```python
from build123d import *

# Parameters (mm, degrees)
F0_R      = 4
F1_DEPTH  = 4
F2_R      = 14.5
F3_DEPTH  = 2
F4_R      = 5
F5_DEPTH  = 1
F3_FACE_R = 14.5
F6_DEPTH  = 2.54


with BuildPart() as f1:
    # F0 (on Top) → F1 (new body)
    with BuildSketch(Plane.XY):
        Circle(F0_R)
    extrude(amount=F1_DEPTH)

    # F2 (on Top) → F3 (join)
    with BuildSketch(Plane.XY):
        Circle(F2_R)
    extrude(amount=-F3_DEPTH)

    # F4 (on Top) → F5 (join)
    with BuildSketch(Plane.XY):
        Circle(F4_R)
    extrude(amount=F5_DEPTH)

    # F3_face (on face) → F6 (join)
    with BuildSketch(Plane(origin=(0, 0, -2), x_dir=(1, 0, 0), z_dir=(0, 0, -1))):
        Circle(F3_FACE_R)
    extrude(amount=F6_DEPTH)


solid = f1.part
```
Build history of the part. All positions in model axes, mm. A direction names the side the tool comes from. Coordinates: 2 decimals unless noted, no trailing zeros. Order: outer loops, then holes, each group sorted by start corner. A loop starts at its lowest first (then second) coordinate and runs counter-clockwise, first axis right, second up. Notation, with made-up numbers: M 73.25,40.5 L 114.25,40.5 A11 cw 114.25,47.5 Z; hole C 66.5,-25.5 d1. An arc over 180 degrees is marked long. One line per question, with ' | ' between items. Start each with the question number.
1. Cut at C-C (z = 1.5). Write the cut outline in (x, y), plus the area to 3 significant figures.
2. Flat gauge pins, fed straight in: P1, Ø2, axis at x = -11, z = -3, coming from the -Y side; P2, Ø3, axis at x = 0.5, z = 2, coming from the +Y side; P3, Ø4, axis at y = 3.5, z = -2, coming from the +X side. Where does each tip first touch, or does it go through?
3. Cut at D-D (x = -6.75). Write the cut outline in (y, z), plus the area to 3 significant figures.
4. Cut at A-A (x = 0). Write the cut outline in (y, z), plus the area to 3 significant figures.
5. Wall check: line 1 along Z through (x, y) = (4.75, 4.5); line 2 along X through (y, z) = (-4.75, -1.75); line 3 along X through (y, z) = (-13, -4). Give the ranges that are in metal, low to high. Write a range as [from, to].
6. Tool access for faces 1 (the face through (-1.08, -4.88, 0.49)), 2 (the face through (0, 0, -4.54)): list every direction of +Z, -Z, +X, -X, +Y, -Y with a clear straight run to the whole face (end or side of a thin tool).
The answers:
1) outline: C 0,0 d8 | area: 50.3 mm2
2) P1: stops at y = -10.5 | P2: stops at y = 5 | P3: stops at x = 14.42
3) outline: M -12.83,-4.54 L 12.83,-4.54 L 12.83,0 L -12.83,0 Z | area: 117 mm2
4) outline: M -14.5,-4.54 L 14.5,-4.54 L 14.5,0 L 5,0 L 5,1 L 4,1 L 4,4 L -4,4 L -4,1 L -5,1 L -5,0 L -14.5,0 Z | area: 166 mm2
5) line 1: z = [-4.54, 0] | line 2: x = [-13.7, 13.7] | line 3: x = [-6.42, 6.42]
6) face 1: +Z | face 2: -Z, +X, -X, +Y, -Y
